Input: part model. Units: mm. Frame: model coordinates. Round coordinates to 2 decimals unless told otherwise and drop trailing zeros. Loops run counter-clockwise (first coordinate to the right, second up) from the corner with the lowest first, then second, coordinate; pieces in that order, holes last. Notation, with made-up numbers: M 79,60 L 117,60 A24 ccw 117,86 Z; hole C 36,69 d9. An arc over 180 degrees is marked long. Put each result on its own line as item: value. Start each with the question number.
1) Pin query (flat end, axial travel): pin 1 (5 mm diameter, centred on x = 29, z = -22.5, fed in from +Y); pin 2 (4 mm diameter, centred on x = -29, z = -22.5, fed in from -Y). Return the tip coordinate at first contact, or that it passes through.
2) Section D-D on y = -4. Output: boundary loops of the cut face in (x, z).
3) Section B-B on z = -22.5. Output: boundary loops of the cut face in (x, y).
4) Draft query along X for faces 1 (the face through (0, -10, -6)), 2 (the face through (1.56, -8.38, 4.96)), 3 (the face through (-35, -5, 0)), 4 (the face through (35, -5, 0)). Return one class per face: +X half, -X half, draft (parallel to the pull), parting line (faces both ways), or undercut.
5) Section C-C on x = 29. Output: boundary loops of the cut face in (y, z).
6) Line query: probe 1 along Z at (x, y) = (-29, -1.75); probe 2 along X at (y, z) = (-3.5, -22.5); probe 3 along X at (y, z) = (-6.75, 22). Output: solid intervals per line, ascending.
7) Section A-A on x = 0. Output: boundary loops of the cut face in (y, z).
from build123d import *

# Parameters (mm, degrees)
SKETCH1_W           = 70
SKETCH1_H           = 55
BOSS_EXTRUDE1_DEPTH = 10
CHAMFER1_SIZE       = 1
SKETCH2_R           = 5.2
CUT_EXTRUDE1_DEPTH  = 46.620718977
CHAMFER2_SIZE       = 1
M5_TAPPED_HOLE1_D   = 4.2


# Read off the part's stored shape, not the designer's step: Draft1
with BuildPart() as part:
    # Sketch1 → Boss-Extrude1 (new body)
    with BuildSketch(Plane(origin=(0, 0, 0), x_dir=(1, 0, 0), z_dir=(0, 1, 0))):
        Rectangle(SKETCH1_W, SKETCH1_H)
    extrude(amount=-BOSS_EXTRUDE1_DEPTH)

    # Chamfer1
    chamfer1_edges = [part.edges().sort_by_distance(p)[0] for p in [
        (-35, -10, 0),
        (0, -10, 27.5),
        (35, -10, 0),
        (0, 0, 27.5),
        (-35, 0, 0),
        (0, 0, -27.5),
        (35, 0, 0),
        (0, -10, -27.5),
    ]]
    chamfer(chamfer1_edges, length=CHAMFER1_SIZE)

    # Sketch2 → Cut-Extrude1 (cut, through all)
    with BuildSketch(Plane(origin=(0, 0, 0), x_dir=(1, 0, 0), z_dir=(0, 1, 0))):
        with Locations(Location((0, 0, 0), (0, 0, 270))):
            Circle(SKETCH2_R)
    extrude(amount=-CUT_EXTRUDE1_DEPTH, mode=Mode.SUBTRACT)

    # Chamfer2
    chamfer2_edges = [part.edges().sort_by_distance(p)[0] for p in [
        (35, -5, -27.5),
        (-35, -5, -27.5),
        (-35, -5, 27.5),
        (35, -5, 27.5),
    ]]
    chamfer(chamfer2_edges, length=CHAMFER2_SIZE)

    # M5 Tapped Hole1 (through all)
    with Locations(Plane(origin=(0, 0, 0), x_dir=(1, 0, 0), z_dir=(0, 1, 0))):
        with Locations((-29, 22.5), (29, 22.5), (29, -22.5), (-29, -22.5)):
            Hole(M5_TAPPED_HOLE1_D / 2)

    # Draft1 outline → Draft1 (revolve, cut)
    with BuildSketch(Plane.XY):
        Polygon((5.2, 0), (5.2, -6.8), (5.675502321, 0), align=None)
    revolve(axis=Axis((0, 0, 0), (0, 1, 0)), mode=Mode.SUBTRACT)


solid = part.part
Geometry results:
1. pin 1: stops at y = 0
1. pin 2: passes through
2. outline: M -35,-26.5 L -34,-27.5 L 34,-27.5 L 35,-26.5 L 35,26.5 L 34,27.5 L -34,27.5 L -35,26.5 Z; hole C -29,-22.5 d4.2; hole C -29,22.5 d4.2; hole C 0,0 d10.79; hole C 29,-22.5 d4.2; hole C 29,22.5 d4.2
3. outline: M -35,-9 L -34,-10 L -31.1,-10 L -31.1,0 L -34,0 L -35,-1 Z; M -26.9,-10 L 26.9,-10 L 26.9,0 L -26.9,0 Z; M 31.1,-10 L 34,-10 L 35,-9 L 35,-1 L 34,0 L 31.1,0 Z
4. face 1: draft
4. face 2: undercut
4. face 3: -X half
4. face 4: +X half
5. outline: M -10,-26.5 L -9,-27.5 L -1,-27.5 L 0,-26.5 L 0,-24.6 L -10,-24.6 Z; M -10,-20.4 L 0,-20.4 L 0,20.4 L -10,20.4 Z; M -10,24.6 L 0,24.6 L 0,26.5 L -1,27.5 L -9,27.5 L -10,26.5 Z
6. probe 1: z = -27.5 to -24.6, -20.4 to 20.4, 24.6 to 27.5
6. probe 2: x = -35 to -31.1, -26.9 to 26.9, 31.1 to 35
6. probe 3: x = -35 to -31.04, -26.96 to 26.96, 31.04 to 35
7. outline: M -10,-26.5 L -9,-27.5 L -1,-27.5 L 0,-26.5 L 0,-5.68 L -6.8,-5.2 L -10,-5.2 Z; M -10,5.2 L -6.8,5.2 L 0,5.68 L 0,26.5 L -1,27.5 L -9,27.5 L -10,26.5 Z
